```python
from build123d import *

# Parameters (mm, degrees)
SKETCH1_W                 = 812.8
SKETCH1_H                 = 77.724
BOSS_EXTRUDE1_DEPTH       = 19.05
SKETCH2_W                 = 71.374
SKETCH2_H                 = 15.875
CUT_EXTRUDE1_DEPTH        = 817.296745672
CUT_EXTRUDE2_REACH        = 818.662
SKETCH3_W                 = 762
SKETCH3_H                 = 11.1125
M8_CLEARANCE_HOLE1_D      = 9.652
M8_CLEARANCE_HOLE1_DEPTH  = 19.05
M2_CLEARANCE_HOLE1_D      = 2.54
M2_CLEARANCE_HOLE1_DEPTH  = 19.05
M25_CLEARANCE_HOLE1_D     = 28.575
M25_CLEARANCE_HOLE1_DEPTH = 19.05
M6_CLEARANCE_HOLE1_D      = 6.7564
M6_CLEARANCE_HOLE1_DEPTH  = 19.05
HOLE1_D                   = 8.128
HOLE1_DEPTH               = 19.05
M5_CLEARANCE_HOLE1_D      = 5.334
M5_CLEARANCE_HOLE1_DEPTH  = 3.175
M5_CLEARANCE_HOLE2_D      = 5.334
M5_CLEARANCE_HOLE2_DEPTH  = 77.724
CHAMFER1_SIZE             = 3.175
FILLET1_R                 = 0.762
FILLET2_R                 = 3.937


with BuildPart() as part:
    # Sketch1 → Boss-Extrude1 (new body)
    with BuildSketch(Plane.XZ.offset(15.875)):
        with Locations((406.4, -34.925)):
            Rectangle(SKETCH1_W, SKETCH1_H)
    extrude(amount=-BOSS_EXTRUDE1_DEPTH)

    # Sketch2 → Cut-Extrude1 (cut, through all)
    with BuildSketch(Plane.ZY):
        with Locations((-34.925, -7.9375)):
            Rectangle(SKETCH2_W, SKETCH2_H)
    extrude(amount=-CUT_EXTRUDE1_DEPTH, mode=Mode.SUBTRACT)

    # Sketch3 → Cut-Extrude2 (cut, up to next)
    with BuildSketch(Plane.XY.offset(3.937), mode=Mode.PRIVATE) as cut_extrude2_sk1:
        with Locations((406.4, -10.31875)):
            Rectangle(SKETCH3_W, SKETCH3_H)
    cut_extrude2_tool1 = extrude(cut_extrude2_sk1.sketch, amount=-CUT_EXTRUDE2_REACH, mode=Mode.PRIVATE) & part.part
    add(cut_extrude2_tool1.solids().sort_by_distance((406.4, -10.31875, 3.937))[0], mode=Mode.SUBTRACT)

    # M8 Clearance Hole1
    with Locations(Plane(origin=(0, 3.175, 0), x_dir=(1, 0, 0), z_dir=(0, 1, 0))):
        with Locations((568.924874752, 19.05), (601.438495912, 19.05), (628.947697627, 19.05), (243.875125248, 19.05), (211.361504088, 19.05), (183.852302373, 19.05), (678.944202666, 20.828), (701.450372003, 20.828), (726.460886343, 20.828), (133.855797334, 20.828), (111.349627997, 20.828), (86.339113657, 20.828)):
            Hole(M8_CLEARANCE_HOLE1_D / 2, depth=M8_CLEARANCE_HOLE1_DEPTH)

    # M2 Clearance Hole1
    with Locations(Plane(origin=(0, 3.175, 0), x_dir=(1, 0, 0), z_dir=(0, 1, 0))):
        with Locations((711.2, 3.175), (711.2, 66.675), (762, 3.175), (762, 66.675), (101.6, 3.175), (50.8, 3.175), (101.6, 66.675), (50.8, 66.675)):
            Hole(M2_CLEARANCE_HOLE1_D / 2, depth=M2_CLEARANCE_HOLE1_DEPTH)

    # M25 Clearance Hole1
    with Locations(Plane(origin=(0, 3.175, 0), x_dir=(1, 0, 0), z_dir=(0, 1, 0))):
        with Locations((664.970837168, 36.83), (147.829162832, 36.83), (406.4, 17.272)):
            Hole(M25_CLEARANCE_HOLE1_D / 2, depth=M25_CLEARANCE_HOLE1_DEPTH)

    # M6 Clearance Hole1
    with Locations(Plane(origin=(0, 3.175, 0), x_dir=(1, 0, 0), z_dir=(0, 1, 0))):
        with Locations((612.775, 10.287), (498.475, 10.287), (314.325, 10.287), (200.025, 10.287), (739.775, 9.525), (690.88, 15.875), (121.92, 15.875), (73.025, 9.525), (647.7, 14.732), (546.1, 14.732), (165.1, 14.732), (266.7, 14.732), (513.925467617, 17.547282407), (298.874532383, 17.547282407)):
            Hole(M6_CLEARANCE_HOLE1_D / 2, depth=M6_CLEARANCE_HOLE1_DEPTH)

    # Hole1
    with Locations(Plane(origin=(0, 3.175, 0), x_dir=(1, 0, 0), z_dir=(0, 1, 0))):
        with Locations((583.538437168, 62.23), (583.538437168, 11.43), (229.261562832, 11.43), (229.261562832, 62.23)):
            Hole(HOLE1_D / 2, depth=HOLE1_DEPTH)

    # M5 Clearance Hole1
    with Locations(Plane(origin=(0, 0, 0.762), x_dir=(-1, 0, 0), z_dir=(0, 0, -1))):
        with Locations((-12.7, -9.525), (-800.1, -9.525)):
            Hole(M5_CLEARANCE_HOLE1_D / 2, depth=M5_CLEARANCE_HOLE1_DEPTH)

    # M5 Clearance Hole2
    with Locations(Plane(origin=(0, 0, -73.787), x_dir=(-1, 0, 0), z_dir=(0, 0, -1))):
        with Locations((-800.1, -9.525), (-774.7, -9.525), (-749.3, -9.525), (-723.9, -9.525), (-698.5, -9.525), (-673.1, -9.525), (-647.7, -9.525), (-622.3, -9.525), (-596.9, -9.525), (-571.5, -9.525), (-546.1, -9.525), (-520.7, -9.525), (-495.3, -9.525), (-469.9, -9.525), (-444.5, -9.525), (-419.1, -9.525), (-393.7, -9.525), (-368.3, -9.525), (-342.9, -9.525), (-317.5, -9.525), (-292.1, -9.525), (-266.7, -9.525), (-241.3, -9.525), (-215.9, -9.525), (-190.5, -9.525), (-165.1, -9.525), (-139.7, -9.525), (-114.3, -9.525), (-88.9, -9.525), (-63.5, -9.525), (-38.1, -9.525), (-12.7, -9.525)):
            Hole(M5_CLEARANCE_HOLE2_D / 2, depth=M5_CLEARANCE_HOLE2_DEPTH)

    # Chamfer1
    chamfer1_edges = [part.edges().sort_by_distance(p)[0] for p in [
        (812.8, -15.875, 2.3495),
        (0, -15.875, -72.1995),
        (787.4, -4.7625, 2.3495),
        (25.4, -4.7625, 2.3495),
        (25.4, -15.875, 2.3495),
        (787.4, -15.875, 2.3495),
        (0, -15.875, 2.3495),
        (812.8, -15.875, -72.1995),
    ]]
    chamfer(chamfer1_edges, length=CHAMFER1_SIZE)

    # Fillet1
    fillet1_edges = [part.edges().sort_by_distance(p)[0] for p in [
        (406.4, 0, -70.612),
        (406.4, 0, 0.762),
    ]]
    fillet(fillet1_edges, radius=FILLET1_R)

    # Fillet2
    fillet2_edges = [part.edges().sort_by_distance(p)[0] for p in [
        (406.4, 3.175, -73.787),
        (406.4, 3.175, 3.937),
    ]]
    fillet(fillet2_edges, radius=FILLET2_R)


solid = part.part
```
The listing builds one solid part. Answer for the finished solid, in the listing's coordinates (mm). A direction names the side the tool comes from. Give positions to 0.01 mm unless a question says otherwise; leave off trailing zeros. Answer in a Markdown table with one row per item. Add a question column.
Q1. Which of the six approach directions +Z, -Z, +X, -X, +Y, -Y give full straight-line access (tool end or side, diameter ignored) to faces 1 (the flat face through (465, -3, 0.762)), 2 (the flat face through (405, -4, 3.937))?
Q2. For a pull along X with two mould halves and no side action, classify faces 3 (the cylindrical face through (679.245, 1.565, -37.458)), 4 (the flat face through (0, 1, -35)), 5 (the flat face through (812.8, 1, -35)) as released by +X, released by -X, zero draft, split by the parting line, or undercut.
Q3. Given P1, Ø12.5, axis at x = 211.36, z = -19.05, coming from the -Y side; P2, Ø4, axis at x = 253.5, y = 1, coming from the -Z side, each flat-ended and moving along its own axis, determine where each tip first touches the part or whether it passes through.
Q4. Find the intervals of material crossed by line 1 along Z through (x, y) = (358, -4.5); line 2 along Z through (x, y) = (514.5, -0.25); line 3 along Z through (x, y) = (770.5, -14.5), in increasing order. Write a range as [from, to].
Determined:
| question | item | result |
|---|---|---|
| 1 | face 1 | +X, -X, -Y |
| 1 | face 2 | +Z, +X, -X, +Y, -Y |
| 2 | face 3 | undercut |
| 2 | face 4 | released by -X |
| 2 | face 5 | released by +X |
| 3 | P1 | stops at y = 0 |
| 3 | P2 | stops at z = -73.79 |
| 4 | line 1 | z = [-73.79, -70.61], [0.76, 3.94] |
| 4 | line 2 | z = [-73.75, -70.41], [0.56, 3.9] |
| 4 | line 3 | z = [-73.79, -70.61] |
